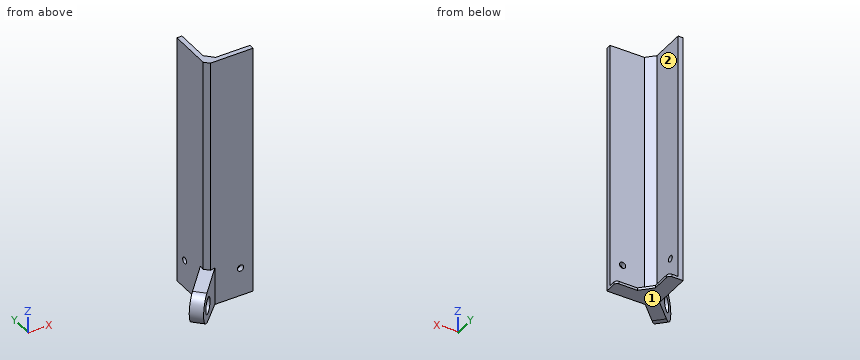
Autodesk Inventor part; units mm, degrees
ref_plane "Work Plane1" through (0, 0, 0) normal (-0.7071, 0.7071, 0) x (0, 0, -1)
ref_plane "YZ Plane" through (0, 0, 0) normal (1, 0, 0) x (0, 1, 0)
ref_plane "XZ Plane" through (0, 0, 0) normal (0, 1, 0) x (-1, 0, 0)
sketch "Sketch1" plane through (0, 0, 0) normal (0, 0, 1) x (1, 0, 0)
  line L0 (1.7958, 0) -> (19.05, 0)
  line L1 (0, 1.7963) -> (0, 19.05)
  line L2 (0, 19.05) -> (2.032, 19.05)
  line L3 (19.05, 0) -> (19.05, 2.032)
  line L4 (0, 1.7963) -> (1.7958, 0)
  line L5 (0, 1.7963) -> (3.81, 1.7963) construction
  line L6 (5.1517, 2.032) -> (19.05, 2.032)
  line L7 (2.032, 5.1527) -> (2.032, 19.05)
  line L8 (2.032, 5.1527) -> (5.1517, 2.032)
  line L9 (19.05, 2.032) -> (2.032, 19.05) construction
  point P0 (0, 0)
  dimension "d0" = 19.05
  dimension "d1" = 19.05
  dimension "d2" = 2.032
  dimension "d3" = 2.032
  dimension "d8" = 3.81
  dimension "d73" = 2.54
  dimension "d74" = 17.2542
extrude "Extrusion1" add sketch "Sketch1" against normal blind 101.6
sketch "Sketch2" plane through (0, 0, -101.6) normal (0, 0, -1) x (-1, 0, 0)
  line L0 (-19.05, 0) -> (-1.7958, 0)
  line L1 (-19.05, 0) -> (-19.05, 5.842)
  line L2 (-19.05, 0) -> (-13.208, 0) construction
  line L3 (-19.05, 5.842) -> (-10.3222, 5.842)
  line L4 (0, 19.05) -> (-2.032, 19.05)
  line L5 (0, 19.05) -> (-5.842, 19.05)
  line L6 (0, 19.05) -> (5.842, 19.05) construction
  line L7 (-5.842, 19.05) -> (-5.842, 10.3222)
  line L8 (-16.4522, -0.288) -> (10.5221, -0.288) construction
  line L9 (0.0018, -0.288) -> (0.2898, 0)
  line L10 (-1.7958, 0) -> (0, 1.7958)
  line L11 (-1.7958, 0) -> (12.0118, 0) construction
  line L12 (-19.05, 0) -> (-1.7958, 0)
  line L13 (0, 1.7958) -> (0, 19.05)
  line L14 (-16.4522, -0.288) -> (-16.1642, 0)
  line L15 (-10.3222, 5.842) -> (-5.842, 10.3222)
  point P0 (0, 0)
  dimension "d11" = 5.842
  dimension "d15" = 5.842
  dimension "d16" = 180
  dimension "d18" = 90
  dimension "d20" = 45
  dimension "d75" = 10.16
extrude "Extrusion2" add sketch "Sketch2" against normal blind 1.016
sketch "Sketch3" plane through (1.7958, 0, 0) normal (-0.7072, -0.707, 0) x (-0.707, 0.7072, 0)
  line L0 (0, 101.6) -> (2.5396, 101.6)
  line L1 (1.7961, 101.6) -> (1.7961, 0) construction
  point P0 (1.2696, 0)
  point P1 (1.7961, 101.6)
ref_plane "Work Plane1" through (0, 0, 0) normal (-0.7071, 0.7071, 0) x (0, 0, -1)
sketch "Sketch5" plane through (0, 0, 0) normal (-0.7071, 0.7071, 0) x (0, 0, -1)
  line L0 (101.6, -13.4704) -> (101.6, -1.2698)
  line L1 (0, -1.2702) -> (101.6, -1.2702)
  line L2 (101.6, -2.5402) -> (86.36, -2.5402)
  line L3 (101.6, -2.5402) -> (116.84, -2.5402) construction
  arc A0 (101.6, 7.6198) -> (89.066, 9.0621) centre (95.25, 7.6198) ccw
  line L4 (101.6, -2.5402) -> (101.6, 7.6198)
  line L5 (86.36, -2.5402) -> (89.066, 9.0621)
  point P0 (0, 0)
  point P1 (95.25, -2.5402)
  dimension "d37" = 1.27
  dimension "d38" = 15.24
  dimension "d39" = 180
  dimension "d40" = 6.35
  dimension "d41" = 10.16
  dimension "d42" = 6.35
  dimension "d43" = 12.7
extrude "Extrusion4" add sketch "Sketch5" along normal mid plane 5.08
sketch "Sketch6" plane through (0, 0, -101.6) normal (0, 0, -1) x (-1, 0, 0)
  point P0 (0, 0)
sketch "Sketch7" plane through (-1.7961, 1.7961, 0) normal (-0.7071, 0.7071, 0) x (-0.7071, -0.7071, 0)
  line L0 (-2.54, -86.36) -> (9.0621, -89.066)
  line L1 (7.6198, -101.6) -> (-2.54, -101.6)
  arc A0 (9.0621, -89.066) -> (7.6198, -101.6) centre (7.6198, -95.25) ccw
  point P0 (0, 0)
  dimension "d46" = 6.35
hole "Hole1" at (-7.1841, -3.592, -95.25) direction (0.7071, -0.7071, 0) diameter 6.35 end through all
fillet "Fillet1" radius 1.27 2 edges at (5.842, 19.05, -101.092) (19.05, 5.842, -101.092)
sketch "Sketch8" plane through (0, 1.7963, 0) normal (-1, 0, 0) x (0, 0, 1)
  line L0 (0, 17.2537) -> (-101.6, 17.2537)
  line L1 (-101.6, 1.7958) -> (-101.6, 17.2537)
  point P0 (0, -1.7963)
  point P1 (-90.17, 12.1737)
  dimension "d55" = 5.08
  dimension "d56" = 11.43
hole "Hole2" at (0, 13.97, -90.17) direction (1, 0, 0) diameter 2.54 end through all
sketch "Sketch9" plane through (1.7958, 0, 0) normal (0, -1, 0) x (1, 0, 0)
  line L0 (17.2542, 0) -> (17.2542, -101.6)
  line L1 (17.2542, -101.6) -> (1.7963, -101.6)
  point P0 (-1.7958, 0)
  point P1 (12.1742, -90.17)
  dimension "d64" = 5.08
  dimension "d65" = 11.43
hole "Hole3" at (13.97, 0, -90.17) direction (0, 1, 0) diameter 2.54 end through all
sketch "Sketch10" plane through (0, 0, 0) normal (0, 0, 1) x (1, 0, 0)
  line L0 (19.05, 2.032) -> (5.1517, 2.032)
  line L1 (2.032, 5.1527) -> (2.032, 19.05)
  line L2 (19.05, 2.032) -> (2.032, 19.05) construction
  point P0 (0, 0)
properties part number "Lopez_CenterLeg"
Geometry: final body of the model. Coordinates: model frame, mm. Face numbers are marked on the shaded views. A direction names the side the tool comes from. Round coordinates to 2 decimals unless told otherwise and drop trailing zeros. Loops run counter-clockwise (first coordinate to the right, second up) from the corner with the lowest first, then second, coordinate; pieces in that order, holes last. Notation, with made-up numbers: (20.25, 85) -> (32.25, 85) arc R30 ccw to (32.25, 121) -> close; hole circle Ø4 at (2, 58). An arc over 180 degrees is marked (long way). Write each question's results on one line, items separated by ' | '.
Item 1: Pin query (flat end, axial travel): pin 1 Ø3 at (y, z) = (4, -21.5) entering from +X; pin 2 Ø12 at (x, z) = (11, -59) entering from -Y; pin 3 Ø1 at (y, z) = (11.5, -78) entering from -X. Return the tip coordinate at first contact, or that it passes through.
Answers below:
pin 1: stops at x = 4.68 | pin 2: stops at y = 0 | pin 3: stops at x = 0
Item 2: Cut plane D-D on z = -90.17. Return the cut outline in (x, y), and give its area (3 significant figures).
Answers below:
outline: (-9.88, -6.29) -> (-6.29, -9.88) -> (3.59, 0) -> (12.7, 0) -> (12.7, 2.03) -> (5.15, 2.03) -> (2.03, 5.15) -> (2.03, 12.7) -> (0, 12.7) -> (0, 3.59) -> close; (0, 15.24) -> (2.03, 15.24) -> (2.03, 19.05) -> (0, 19.05) -> close; (15.24, 0) -> (19.05, 0) -> (19.05, 2.03) -> (15.24, 2.03) -> close | area: 132 mm²
Item 3: Cut plane C-C on y = 11.5. Return the cut outline in (x, z).
Answers below:
outline: (0, -101.6) -> (5.84, -101.6) -> (5.84, -100.58) -> (2.03, -100.58) -> (2.03, 0) -> (0, 0) -> close
Item 4: Line query: probe 1 along Z at (x, y) = (13.97, 0.4); probe 2 along Y at (x, z) = (9.5, -9). Output: solid intervals per line, ascending. Write a range as [from, to].
Answers below:
probe 1: z = [-101.6, -91.44], [-88.9, 0] | probe 2: y = [0, 2.03]
Item 5: Set-up query: the marked faces 1 and 2. Return all of +Z, -Z, +X, -X, +Y, -Y with unobstructed straight access to the full face (end or side cutting, diameter ignored); none if empty.
Answers below:
face 1: -Z, +X, -X, +Y, -Y | face 2: +Z, +X, +Y
Item 6: Cut plane B-B on z = -80. Return the cut outline in (x, y), and give its area (3 significant figures).
Answers below:
outline: (0, 1.8) -> (1.8, 0) -> (19.05, 0) -> (19.05, 2.03) -> (5.15, 2.03) -> (2.03, 5.15) -> (2.03, 19.05) -> (0, 19.05) -> close | area: 76.5 mm²
Item 7: Cut plane A-A on x = 13.97. Return the cut outline in (y, z).
Answers below:
outline: (0, -101.6) -> (5.84, -101.6) -> (5.84, -100.58) -> (2.03, -100.58) -> (2.03, -91.44) -> (0, -91.44) -> close; (0, -88.9) -> (2.03, -88.9) -> (2.03, 0) -> (0, 0) -> close
